Can you work these out from the drawing? Everything is in mm from the part's minimum corner. A direction names the side the tool comes from. Give positions to 0.01 mm unless a question says otherwise; leave off trailing zeros. Write each loop counter-clockwise with the first axis right and the second up, starting at its lowest first coordinate (ties: lowest second). Pieces come first, ordered by that corner, then holes. Notation, with made-up numbers: M 4,27 L 39,27 A13 cw 39,40 Z; hole C 65.25,64.25 d2. An arc over 180 degrees is marked long. One line per item, written item: value.
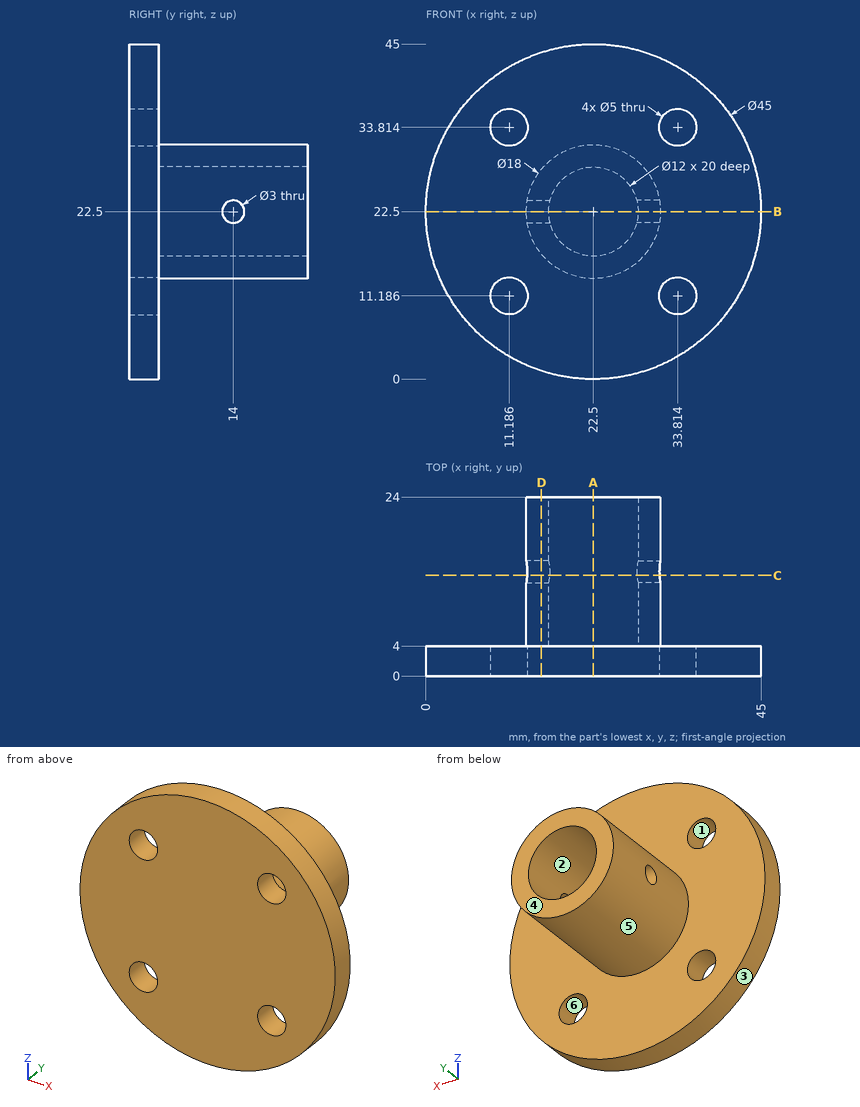
1) If we section it at B-B, the plane z = 22.5: Write out the boundary of the cut face in (x, y).
Outcome:
outline: M 0,0 L 45,0 L 45,4 L 31.5,4 L 31.5,12.5 L 28.5,12.5 L 28.5,4 L 16.5,4 L 16.5,12.5 L 13.5,12.5 L 13.5,4 L 0,4 Z; M 13.5,15.5 L 16.5,15.5 L 16.5,24 L 13.5,24 Z; M 28.5,15.5 L 31.5,15.5 L 31.5,24 L 28.5,24 Z
2) I'm going to push flat-ended pins straight in: pin 1 (4.5 mm diameter, centred on x = 33.81, z = 11.19, fed in from +Y); pin 2 (3 mm diameter, centred on y = 4.5, z = 14.5, fed in from +X) (1 decimal); pin 3 (5 mm diameter, centred on x = 14, y = 17, fed in from -Z); pin 4 (12 mm diameter, centred on x = 32, y = 8.5, fed in from -Z). Where does each tip first touch, or does it pass through?
Outcome:
pin 1: passes through
pin 2: stops at x = 44
pin 3: stops at z = 15.79
pin 4: stops at z = 0.69
3) On a 3-axis mill with a long thin cutter (end or side, diameter ignored), from which of +Z, -Z, +X, -X, +Y, -Y can I reach the whole of each face in a straight line? I mean the marked faces 5 and 6. Say none if no direction works.
Outcome:
face 5: +Y
face 6: +Y, -Y
4) If we section it at C-C, the plane y = 13.5: Write out the boundary of the cut face in (x, z).
Outcome:
outline: M 13.61,21.09 A9 ccw 31.39,21.09 L 28.33,21.09 A6 cw 16.67,21.09 Z; M 13.61,23.91 L 16.67,23.91 A6 cw 28.33,23.91 L 31.39,23.91 A9 ccw Z
5) We'd pull the mould along X, two halves only. Please class the marked faces 1, 2, 3 and 4: pulls with the +X half, pulls with the -X half, needs draft (parallel to the pull), parting line crosses it, or undercut.
Outcome:
face 1: undercut
face 2: undercut
face 3: parting line crosses it
face 4: needs draft
6) If we section it at D-D, the plane x = 15.5: Write out the boundary of the cut face in (y, z).
Outcome:
outline: M 0,1.12 L 4,1.12 L 4,16.84 L 24,16.84 L 24,28.16 L 4,28.16 L 4,43.88 L 0,43.88 Z; hole C 14,22.5 d3
7) Please list where these lines run through material, in increasing order: L1, parallel to X at y = 3.25, z = 11; L2, parallel to Y at x = 10.5, z = 6.5; L3, parallel to Z at x = 20, y = 10.5 (1 decimal). Write a range as from..to.
Outcome:
L1: x = 3.16..8.69, 13.68..31.32, 36.31..41.84
L2: y = 0..4
L3: z = 13.9..17, 28..31.1
8) If we section it at A-A, the plane x = 22.5: Write out the boundary of the cut face in (y, z), then the cut area to 3 significant figures.
Outcome:
outline: M 0,0 L 4,0 L 4,13.5 L 24,13.5 L 24,16.5 L 4,16.5 L 4,28.5 L 24,28.5 L 24,31.5 L 4,31.5 L 4,45 L 0,45 Z
area: 300 mm^2
